Could you check a few things on this model? Use its own coordinates, in mm. A direction names the side the tool comes from. Coordinates: 2 decimals unless noted, no trailing zeros. Loops run counter-clockwise (first coordinate to the right, second up) from the corner with the lowest first, then second, coordinate; pieces in that order, holes last. Notation, with made-up numbers: (27, -17.75) - (38, -17.75) arc R27 ccw to (38, 11.25) - close; hole circle Ø6 at (1.5, 37). An arc over 180 degrees is marked (long way). One line per item, written item: value. Start each with the question number.
(1) If we mould it in two halves opening along Y, with no side actions, what happens to faces 6 (the face through (37, -0.001, -21)), 7 (the face through (-55, 16.7, -21.4)), 8 (the face through (-49.82, 21.68, -20.64)), 9 (the face through (-10, 25.139, -112))? For each: pulls with the +Y half, pulls with the -Y half, needs draft (parallel to the pull), parting line crosses it, or undercut.
(2) If we section it at A-A on y = 6.5: Write out the boundary of the cut face in (x, z), then the cut area to 3 significant figures.
(3) If we section it at D-D on z = -7.5: Count the separate pieces of the cut face and the enclosed holes in it, then the cut area to 3 significant figures.
(4) On a 3-axis mill with a long thin cutter (end or side, diameter ignored), from which of +Z, -Z, +X, -X, +Y, -Y can I reach the whole of each face in a straight line? I mean faces 1 (the face through (28.68, 21.68, -20.64)), 2 (the face through (-9.75, 22.4, 68.95)), 3 (the face through (37, 3, -21)), 4 (the face through (-57, -0.001, -21)), 5 (the face through (-10, 13, -116.044)). Say none if no direction works.
(5) If we section it at B-B on x = -6.5: Write out the boundary of the cut face in (y, z).
(6) I'm going to push flat-ended pins straight in: P1, Ø8, axis at y = 10.5, z = -37.5, coming from the -X side; P2, Ø2.5, axis at x = 36.5, z = -10.5, coming from the +Y side; P3, Ø12.5, axis at y = 14.5, z = -15, coming from the +X side. Where does each tip first touch, or does it pass through?
(7) If I drill on line 1 along X through (y, z) = (2.5, -25.5); line 2 along Z through (x, y) = (-10.5, 8); line 3 along X through (y, z) = (11, -59.5), over which ranges is the centre line in solid material (lowest first)? Write a range as from..to.
```python
from build123d import *

# Parameters (mm, degrees)
SKETCH1_W                = 89
SKETCH1_H                = 192
BOSS_EXTRUDE1_DEPTH      = 30
SKETCH2_R                = 34.99943994
CUT_EXTRUDE1_DEPTH       = 10
SKETCH3_W                = 75
SKETCH3_H                = 5
CUT_EXTRUDE2_DEPTH       = 102
CUT_EXTRUDE4_DEPTH       = 102
SKETCH6_W                = 10.5
SKETCH6_H                = 4
CUT_EXTRUDE7_DEPTH       = 8
BOSS_EXTRUDE2_DEPTH      = 10.5
CUT_EXTRUDE8_DEPTH       = 20.767757578
BOSS_EXTRUDE3_DEPTH      = 10.5
CUT_EXTRUDE9_DEPTH       = 22.812544275
BOSS_EXTRUDE6_DEPTH      = 10.5
BOSS_EXTRUDE7_DEPTH      = 10.5
FILLET1_R                = 10
FILLET2_R                = 10
FILLET3_R                = 10
FILLET4_R                = 10
CUT_EXTRUDE11_DEPTH      = 99
SKETCH15_W               = 7.554212703
SKETCH15_H               = 3.259234926
CUT_EXTRUDE12_DEPTH      = 99
FILLET5_R                = 10
BOSS_EXTRUDE8_DEPTH      = 0.001
BOSS_EXTRUDE8_DEPTH_BACK = 3
SKETCH16_W               = 5
SKETCH16_H               = 192


with BuildPart() as part:
    # Sketch1 → Boss-Extrude1 (new body)
    with BuildSketch(Plane(origin=(0, 0, 0), x_dir=(1, 0, 0), z_dir=(0, 1, 0))):
        with Locations((-10.5, 20.043668932)):
            Rectangle(SKETCH1_W, SKETCH1_H)
        with BuildLine():
            Line((-44.5, -34.956331068), (-44.5, 75.043668932))
            ThreePointArc((-44.5, 75.043668932), (-10.5, 109.043668932), (23.5, 75.043668932))
            Line((23.5, 75.043668932), (23.5, -34.956331068))
            ThreePointArc((23.5, -34.956331068), (-10.5, -68.956331068), (-44.5, -34.956331068))
        make_face(mode=Mode.SUBTRACT)
    extrude(amount=BOSS_EXTRUDE1_DEPTH)

    # Sketch2 → Cut-Extrude1 (cut)
    with BuildSketch(Plane.XZ):
        with Locations((-10.5, 37.838844027)):
            Circle(SKETCH2_R)
    extrude(amount=-CUT_EXTRUDE1_DEPTH, mode=Mode.SUBTRACT)

    # Sketch3 → Cut-Extrude2 (cut)
    with BuildSketch(Plane(origin=(34, 0, 0), x_dir=(0, 0, -1), z_dir=(1, 0, 0))):
        with Locations((-34.286288065, 12.5)):
            Rectangle(SKETCH3_W, SKETCH3_H)
    extrude(amount=-CUT_EXTRUDE2_DEPTH, mode=Mode.SUBTRACT)

    # Sketch4 → Cut-Extrude4 (cut)
    with BuildSketch(Plane.ZY.offset(55)):
        Polygon((-40.970715348, 29.469395922), (-41.211628541, 24.561719678), (-3.213711935, 10), (-3.213711935, 15), align=None)
    extrude(amount=-CUT_EXTRUDE4_DEPTH, mode=Mode.SUBTRACT)

    # Sketch6 → Cut-Extrude7 (cut)
    with BuildSketch(Plane(origin=(0, 30, 0), x_dir=(1, 0, 0), z_dir=(0, 1, 0))):
        with Locations((-49.75, 40.570603007)):
            Rectangle(SKETCH6_W, SKETCH6_H)
        with Locations((28.75, 40.570603007)):
            Rectangle(SKETCH6_W, SKETCH6_H)
    extrude(amount=-CUT_EXTRUDE7_DEPTH, mode=Mode.SUBTRACT)

    # Sketch7 → Boss-Extrude2 (add)
    with BuildSketch(Plane.ZY.offset(55)):
        Polygon((-38.570603007, 23.549614886), (-42.570603007, 25.082511526), (-42.570603007, 22), (-38.570603007, 22), align=None)
    extrude(amount=-BOSS_EXTRUDE2_DEPTH)

    # Sketch8 → Cut-Extrude8 (cut)
    with BuildSketch(Plane.ZY.offset(55)):
        Polygon((-42.570603007, 25.082511526), (-55.402488324, 30), (-42.570603007, 30), align=None)
    extrude(amount=-CUT_EXTRUDE8_DEPTH, mode=Mode.SUBTRACT)

    # Sketch9 → Boss-Extrude3 (add)
    with BuildSketch(Plane(origin=(34, 0, 0), x_dir=(0, 0, -1), z_dir=(1, 0, 0))):
        Polygon((38.570603007, 23.549614886), (42.570603007, 25.082511526), (42.570603007, 22), (38.570603007, 22), align=None)
    extrude(amount=-BOSS_EXTRUDE3_DEPTH)

    # Sketch10 → Cut-Extrude9 (cut)
    with BuildSketch(Plane(origin=(34, 0, 0), x_dir=(0, 0, -1), z_dir=(1, 0, 0))):
        Polygon((42.570603007, 25.082511526), (55.402488324, 30), (42.570603007, 30), align=None)
    extrude(amount=-CUT_EXTRUDE9_DEPTH, mode=Mode.SUBTRACT)

    # Sketch12 → Boss-Extrude6 (add)
    with BuildSketch(Plane.ZY.offset(55)):
        Polygon((-38.570603007, 30), (-41.570603007, 30), (-38.570603007, 28.549614886), align=None)
    extrude(amount=-BOSS_EXTRUDE6_DEPTH)

    # Sketch11 → Boss-Extrude7 (add)
    with BuildSketch(Plane(origin=(34, 0, 0), x_dir=(0, 0, -1), z_dir=(1, 0, 0))):
        Polygon((38.570603007, 28.549614886), (41.570603007, 30.007074027), (38.570603007, 30), align=None)
    extrude(amount=-BOSS_EXTRUDE7_DEPTH)

    # Fillet1
    fillet1_edges = [part.edges().sort_by_distance(p)[0] for p in [
        (-49.75, 30, -55.402488324),
    ]]
    fillet(fillet1_edges, radius=FILLET1_R)

    # Fillet2
    fillet2_edges = [part.edges().sort_by_distance(p)[0] for p in [
        (28.75, 30, -55.402488324),
    ]]
    fillet(fillet2_edges, radius=FILLET2_R)

    # Fillet3
    fillet3_edges = [part.edges().sort_by_distance(p)[0] for p in [
        (-49.75, 10, -3.213711935),
    ]]
    fillet(fillet3_edges, radius=FILLET3_R)

    # Fillet4
    fillet4_edges = [part.edges().sort_by_distance(p)[0] for p in [
        (28.75, 10, -3.213711935),
    ]]
    fillet(fillet4_edges, radius=FILLET4_R)

    # Sketch14 → Cut-Extrude11 (cut)
    with BuildSketch(Plane(origin=(34, 0, 0), x_dir=(0, 0, -1), z_dir=(1, 0, 0))):
        Polygon((42.717415751, 25.138773717), (116.043668932, 25.138773717), (116.043668932, 30), (57.252994033, 30), (53.674522762, 29.337801849), align=None)
    extrude(amount=-CUT_EXTRUDE11_DEPTH, mode=Mode.SUBTRACT)


with BuildPart() as cut_extrude11_piece_1:
    # of the separate pieces the step leaves, piece 1, a body of its own (cut_extrude11_pieces)
    add(part.part.solids().sort_by_distance((23.5, 25.138773717, -42.717415751))[0])

    # Fillet5
    fillet5_edges = [cut_extrude11_piece_1.edges().sort_by_distance(p)[0] for p in [
        (-49.75, 25.138773717, -42.717415751),
        (28.75, 25.138773717, -42.717415751),
    ]]
    fillet(fillet5_edges, radius=FILLET5_R)

    # Sketch16 → Boss-Extrude8 (add, two sides: drawn at the far end of the back side and taken through both)
    with BuildSketch(Plane(origin=(0, 0, 0), x_dir=(-1, 0, 0), z_dir=(0, -1, 0)).offset(-BOSS_EXTRUDE8_DEPTH_BACK)):
        with Locations((-36.5, 20.043668932)):
            Rectangle(SKETCH16_W, SKETCH16_H)
        with Locations((57.5, 20.043668932)):
            Rectangle(SKETCH16_W, SKETCH16_H)
    extrude(amount=BOSS_EXTRUDE8_DEPTH + BOSS_EXTRUDE8_DEPTH_BACK)


with BuildPart() as cut_extrude11_piece_2:
    # of the separate pieces the step leaves, piece 2, a body of its own (cut_extrude11_pieces)
    add(part.part.solids().sort_by_distance((23.5, 30, -57.252994033))[0])


with BuildPart() as cut_extrude11_piece_3:
    # of the separate pieces the step leaves, piece 3, a body of its own (cut_extrude11_pieces)
    add(part.part.solids().sort_by_distance((-55, 30, -57.252994033))[0])


with BuildPart() as cut_extrude12_tool:
    # Sketch15 → Cut-Extrude12 (new body)
    with BuildSketch(Plane(origin=(34, 0, 0), x_dir=(0, 0, -1), z_dir=(1, 0, 0))):
        with Locations((54.846987071, 29.864387296)):
            Rectangle(SKETCH15_W, SKETCH15_H)
    extrude(amount=-CUT_EXTRUDE12_DEPTH)


with BuildPart() as cut_extrude11_piece_2_1:
    add(cut_extrude11_piece_2.part)

    # Cut-Extrude12: cut by cut_extrude12_tool
    add(cut_extrude12_tool.part, mode=Mode.SUBTRACT)


with BuildPart() as cut_extrude11_piece_3_1:
    add(cut_extrude11_piece_3.part)

    # Cut-Extrude12: cut by cut_extrude12_tool
    add(cut_extrude12_tool.part, mode=Mode.SUBTRACT)


solid = cut_extrude11_piece_1.part
```
Values:
1. face 6: pulls with the -Y half
1. face 7: needs draft
1. face 8: undercut
1. face 9: pulls with the +Y half
2. outline: (-55, -116.04) - (34, -116.04) - (34, 75.96) - (-55, 75.96) - close; hole (-44.5, -75.04) arc R34 ccw to (23.5, -75.04) - (23.5, 29.53) arc R35 ccw (long way) to (-44.5, 29.53) - close
2. area: 5,660 mm2
3. separate pieces: 4
3. enclosed holes: 0
3. area: 555 mm2
4. face 1: +X, -X
4. face 2: +Y, -Y
4. face 3: +Z, -Z, +X, +Y
4. face 4: +Z, -Z, +X, -X, -Y
4. face 5: -Z, +X, -X, +Y, -Y
5. outline: (0, -116.04) - (25.14, -116.04) - (25.14, -108.81) - (0, -108.81) - close; (0, 72.61) - (10, 72.61) - (10, 71.79) - (15, 71.79) - (15, 68.72) - (30, 68.72) - (30, 75.96) - (0, 75.96) - close
6. P1: stops at x = -55
6. P2: stops at y = 3
6. P3: stops at x = 34
7. line 1: x = -60..-44.5, 23.5..39
7. line 2: z = -116.04..-109.04, 72.84..75.96
7. line 3: x = -55..-44.5, 23.5..34
